For this review, use the dimensioned drawing (mm, ordinates from the lowest corner) and the shaded views. Give positions to 0.01 mm unless a question says otherwise; leave off trailing zeros. Loops run counter-clockwise (first coordinate to the right, second up) from the corner with the lowest first, then second, coordinate; pieces in that order, holes last. Notation, with made-up numbers: (14.25, 81) -> (51.25, 81) arc R16 cw to (51.25, 109) -> close; hole circle Ø11 at (-2.75, 40.5). An arc over 180 degrees is marked (long way). Write each question's results on one line, items separated by ' | '. Start each with the question number.
Q1. Insertion check: pin 1 Ø2 at (x, y) = (3.18, 2.75) entering from -Z. The pin has a flat end and moves straight along its axis. Give the tip position at first contact, or say it passes through.
Q2. Wall thickness on L1, parallel to Y at x = 3.25, z = 1.5; L2, parallel to Y at x = 3.25, z = 10.25; L3, parallel to Z at x = 3.25, y = 1.1: over which ranges is each line inside the solid? List them lowest first. Write a range as [from, to].
Q3. Mouldability with a two-part tool opening along Y and no side actions: class the marked faces 1, 2 and 3 as released by +Y, released by -Y, zero draft, split by the parting line, or undercut.
Q4. We need section D-D (y = 0.55). Write out the cut boundary in (x, z).
Q5. We need section C-C (x = 2.5). Write out the cut boundary in (y, z).
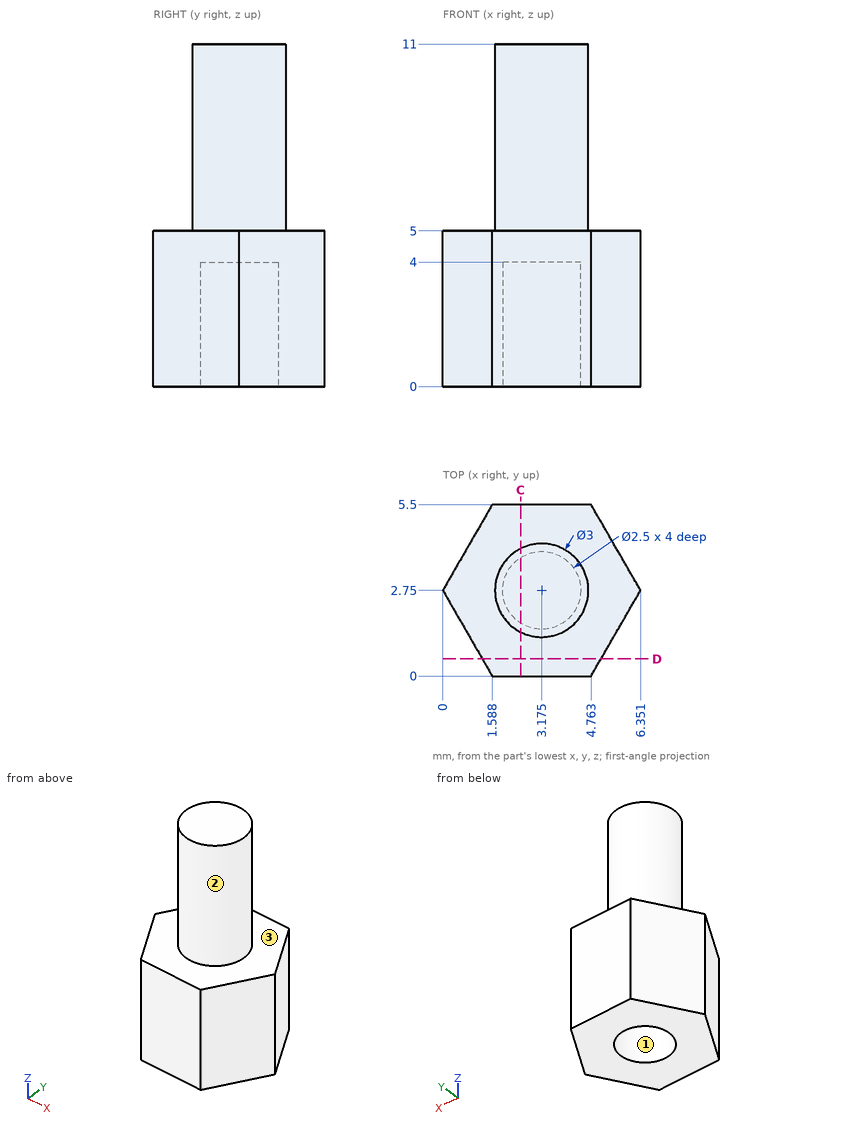
Output:
1) pin 1: z = 4
2) L1: [0, 1.5], [4, 5.5] | L2: [1.25, 4.25] | L3: [0, 5]
3) face 1: undercut | face 2: split by the parting line | face 3: zero draft
4) outline: (1.27, 0) -> (5.08, 0) -> (5.08, 5) -> (1.27, 5) -> close
5) outline: (0, 0) -> (1.7, 0) -> (1.7, 4) -> (3.8, 4) -> (3.8, 0) -> (5.5, 0) -> (5.5, 5) -> (4.09, 5) -> (4.09, 11) -> (1.41, 11) -> (1.41, 5) -> (0, 5) -> close
